Autodesk Inventor part; units mm, degrees
ref_plane "Start Plane" through (0, 0, 0) normal (0, 0, 1) x (1, 0, 0)
ref_plane "End Plane" through (0, 0, 1500) normal (0, 0, 1) x (1, 0, 0)
ref_plane "YZ Plane" through (0, 0, 0) normal (1, 0, 0) x (0, 1, 0)
ref_plane "Start Plane" through (0, 0, 0) normal (0, 0, 1) x (1, 0, 0)
ref_plane "End Plane" through (0, 0, 1500) normal (0, 0, 1) x (1, 0, 0)
sketch "Sketch" plane through (0, 0, 0) normal (0, 0, 1) x (1, 0, 0)
  line L0 (-85, 167.3) -> (-22, 167.3)
  line L1 (-85, 180) -> (-85, 167.3)
  line L2 (85, 180) -> (-85, 180)
  line L3 (85, 167.3) -> (85, 180)
  line L4 (22, 167.3) -> (85, 167.3)
  line L5 (4, -149.3) -> (4, 149.3)
  line L6 (85, -167.3) -> (22, -167.3)
  line L7 (85, -180) -> (85, -167.3)
  line L8 (-85, -167.3) -> (-85, -180)
  line L9 (-22, -167.3) -> (-85, -167.3)
  line L10 (-4, 149.3) -> (-4, -149.3)
  line L11 (0, -252) -> (0, 252) construction
  line L12 (-4, -167.3) -> (4, -167.3) construction
  arc A0 (-22, -167.3) -> (-4, -149.3) centre (-22, -149.3) ccw
  arc A1 (-4, 149.3) -> (-22, 167.3) centre (-22, 149.3) ccw
  arc A2 (22, 167.3) -> (4, 149.3) centre (22, 149.3) ccw
  arc A3 (4, -149.3) -> (22, -167.3) centre (22, -149.3) ccw
  line L13 (-119, 0) -> (119, 0) construction
  line L14 (-85, -180) -> (85, -180)
  point P0 (-4, 167.3)
  point P1 (4, 167.3)
  point P2 (0, 0)
  point P3 (0, -167.3)
  point P4 (0, 0)
  dimension "d1" = 360
  dimension "d3" = 12.7
  dimension "d5" = 8
  dimension "d7" = 170
  dimension "d13" = 18
  dimension "d14" = 180
  dimension "d15" = 85
extrude "Body" add sketch "Sketch" along normal up to surface (1500 mm away) from surface at 0
sketch "Sketch3" plane through (0, 0, 0) normal (0, 0, 1) x (1, 0, 0)
  line L0 (0, 0) -> (10, 0)
ref_plane "Work Plane3" through (0, 0, 0) normal (0, -1, 0) x (1, 0, 0)
sketch "Sketch4" plane through (0, 0, 0) normal (0, -1, 0) x (1, 0, 0)
  line L0 (-2, 0) -> (12, 0)
  line L1 (-2, 1500) -> (12, 1500)
  dimension "d19" = 1500
equation "\"d1\" = ParH"
equation "\"d3\" = t2"
equation "\"d7\" = b"
equation "\"d13\" = R1"
equation "\"d14\" = 0.5 * d1"
equation "\"d15\" = 0.5 * d7"
equation "\"d8\" = G_L"
equation "\"b\" = 170"
equation "\"ParH\" = 360"
equation "\"R1\" = 18"
equation "\"G_L\" = d19"
equation "\"t1\" = 8"
equation "\"t2\" = 12.7"
equation "\"G_OFFSET_START\" = 0"
equation "\"G_OFFSET_END\" = 0"
properties part number "DIN 1025 - IPE 360-1500" material "Steel, Mild"
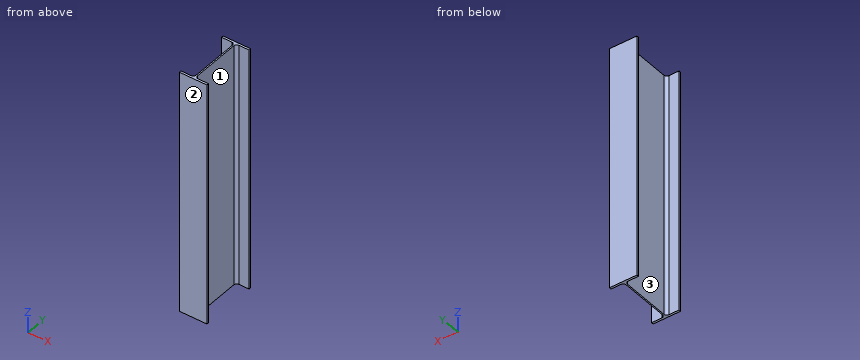
Could you check a few things on this model? Use its own coordinates, in mm. Face numbers are marked on the shaded views. A direction names the side the tool comes from. Give positions to 0.01 mm unless a question says otherwise; leave off trailing zeros. Loops run counter-clockwise (first coordinate to the right, second up) from the corner with the lowest first, then second, coordinate; pieces in that order, holes last. Notation, with made-up numbers: (80.5, -2) -> (103.5, -2) arc R22 cw to (103.5, 6) -> close; hole circle Ø10 at (77, 4.5). An arc over 180 degrees is marked (long way). Answer as CSV lines item,"result". Start each with the question number.
(1) I need wall thicknesses on probe 1 along Y at (x, z) = (62, 689.5); probe 2 along Y at (x, z) = (-20, 1032); probe 3 along X at (y, z) = (-130, 1405.5). Which ranges of each line are inside material? Lowest first, please.
(2) Which directions (+Z, -Z, +X, -X, +Y, -Y) give clear straight access to the entire face, cutting with the end or side of a thin tool? Please do the marked faces 1, 2 and 3.
(3) I'm going to push flat-ended pins straight in: pin 1 Ø10 at (x, y) = (11.5, 83.5) entering from -Z; pin 2 Ø2 at (y, z) = (39, 1194.5) entering from -X; pin 3 Ø1 at (y, z) = (-107, 227) entering from +X. Where does each tip first touch, or does it pass through?
(4) If we section it at C-C on y = 116: Write out the boundary of the cut face in (x, z).
(5) If we section it at B-B on z = 135: Write out the boundary of the cut face in (x, y).
(6) If we section it at A-A on x = -42: Write out the boundary of the cut face in (y, z), then the cut area to 3 significant figures.
Computed:
1,probe 1,"y = -180 to -167.3, 167.3 to 180"
1,probe 2,"y = -180 to -167.19, 167.19 to 180"
1,probe 3,"x = -4 to 4"
2,face 1,"+Z, -Z, +X"
2,face 2,"+Z, -Z, +X, -X, -Y"
2,face 3,"+Z, -Z, -X"
3,pin 1,"passes through"
3,pin 2,"stops at x = -4"
3,pin 3,"stops at x = 4"
4,outline,"(-4, 0) -> (4, 0) -> (4, 1500) -> (-4, 1500) -> close"
5,outline,"(-85, -180) -> (85, -180) -> (85, -167.3) -> (22, -167.3) arc R18 cw to (4, -149.3) -> (4, 149.3) arc R18 cw to (22, 167.3) -> (85, 167.3) -> (85, 180) -> (-85, 180) -> (-85, 167.3) -> (-22, 167.3) arc R18 cw to (-4, 149.3) -> (-4, -149.3) arc R18 cw to (-22, -167.3) -> (-85, -167.3) -> close"
6,outline,"(-180, 0) -> (-167.3, 0) -> (-167.3, 1500) -> (-180, 1500) -> close; (167.3, 0) -> (180, 0) -> (180, 1500) -> (167.3, 1500) -> close"
6,area,"38,100 mm2"
